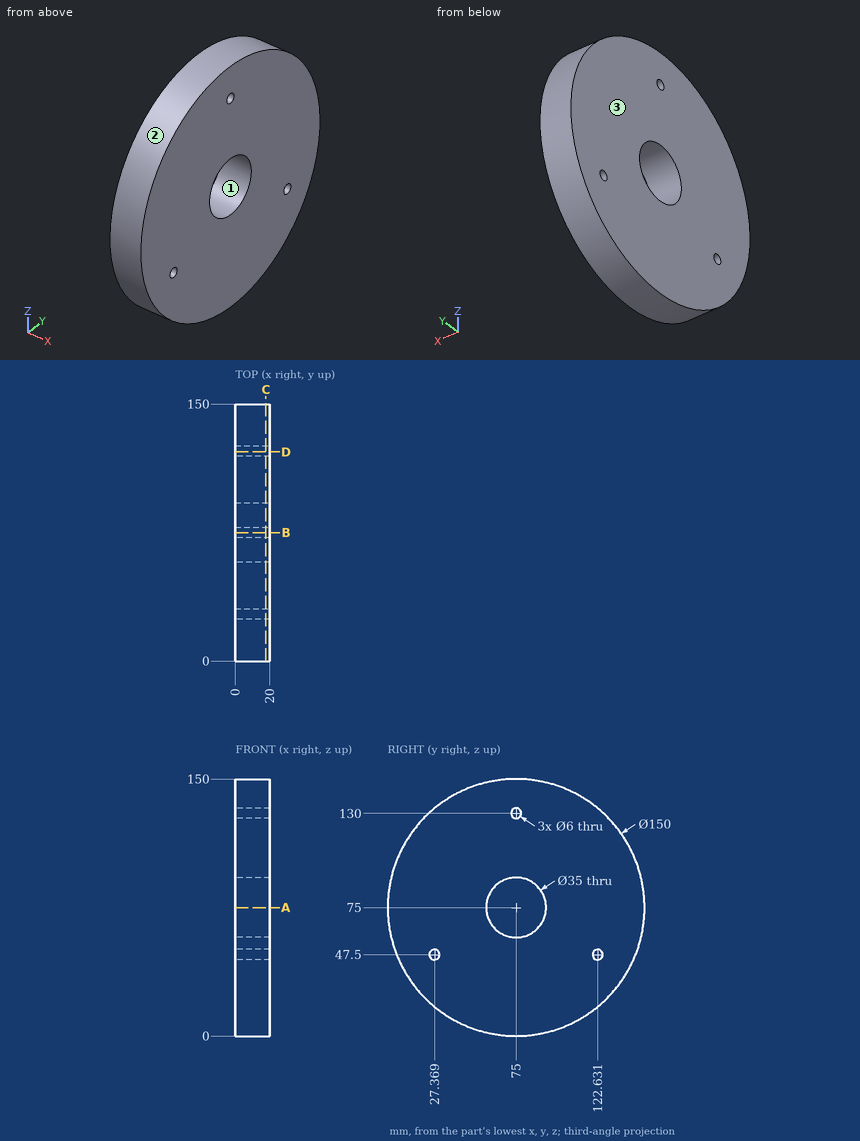
Design review of the part shown in the three views and the two pictorial views. Dimensions are in mm from the part's minimum x, y and z. Coordinates: 2 decimals unless noted, no trailing zeros. Loops run counter-clockwise (first coordinate to the right, second up) from the corner with the lowest first, then second, coordinate; pieces in that order, holes last.
Q1. We need section B-B on y = 75. State the section outline as (x, z) points, and give its area (3 significant figures).
Reported:
outline: (0, 0) - (20, 0) - (20, 57.5) - (0, 57.5) - close; (0, 92.5) - (20, 92.5) - (20, 127) - (0, 127) - close; (0, 133) - (20, 133) - (20, 150) - (0, 150) - close
area: 2,180 mm2
Q2. To check wall thickness, follow line 1 (Y direction, x = 3, z = 86); line 2 (Y direction, x = 9.75, z = 60.5) (1 decimal); line 3 (Z direction, x = 19, y = 82). State the ranges of each line that lie inside material, in increasing order.
Reported:
line 1: y = 0.81 to 61.39, 88.61 to 149.19
line 2: y = 1.4 to 65.2, 84.8 to 148.6
line 3: z = 0.33 to 58.96, 91.04 to 149.67
Q3. The part is to be moulded in two halves that separate along Y. For the marked faces 1, 2 and 3, say which applies: +Y half, -Y half, draft (parallel to the pull), parting line (faces both ways), or undercut.
Reported:
face 1: undercut
face 2: parting line
face 3: draft
Q4. We need section A-A on z = 75. State the section outline as (x, y) points.
Reported:
outline: (0, 0) - (20, 0) - (20, 57.5) - (0, 57.5) - close; (0, 92.5) - (20, 92.5) - (20, 150) - (0, 150) - close
Q5. For pin 1 (6 mm diameter, centred on x = 15, z = 70, fed in from -Y); pin 2 (1 mm diameter, centred on x = 4.5, z = 82, fed in from +Y); pin 3 (5 mm diameter, centred on x = 10, z = 34, fed in from -Y) (1 decimal), all flat-tipped, find the tip position at first contact; note any pin that passes through.
Reported:
pin 1: stops at y = 0.03
pin 2: stops at y = 149.72
pin 3: stops at y = 10.6
Q6. We need section D-D on y = 122. State the section outline as (x, z) points.
Reported:
outline: (0, 16.55) - (20, 16.55) - (20, 44.57) - (0, 44.57) - close; (0, 50.43) - (20, 50.43) - (20, 133.45) - (0, 133.45) - close
Q7. We need section C-C on x = 17.75. State the section outline as (y, z) points.
Reported:
outline: circle Ø150 at (75, 75); hole circle Ø6 at (27.37, 47.5); hole circle Ø35 at (75, 75); hole circle Ø6 at (75, 130); hole circle Ø6 at (122.63, 47.5)
